from build123d import *

# Parameters (mm, degrees)
SKETCH2_R           = 0.635
BOSS_EXTRUDE1_DEPTH = 4.5
CIRPATTERN1_COUNT   = 4
CIRPATTERN1_ANGLE   = 216


with BuildPart() as part:
    # Sketch1 → Revolve1 (revolve)
    with BuildSketch(Plane.XY, mode=Mode.PRIVATE) as revolve1_sk:
        Polygon((0, 0), (7.6, 0), (7.6, -2.3), (6.375, -2.3), (6.375, -15.8), (5.728350463, -15.8), (5.728350463, -20.8), (0, -20.8), align=None)
    revolve(revolve1_sk.sketch.rotate(Axis((0, -20.8, 0), (0, 1, 0)), 90), axis=Axis((0, -20.8, 0), (0, 1, 0)))

    # Sketch2 → Boss-Extrude1 (add)
    with BuildSketch(Plane.XZ.offset(20.8)):
        with Locations(Location((0, 3.773128742, 0), (0, 0, 270))):
            Circle(SKETCH2_R)
    boss_extrude1 = extrude(amount=BOSS_EXTRUDE1_DEPTH)

    # CirPattern1: Boss-Extrude1 ×4 about axis
    cirpattern1_axis = Axis((0, 0, 0), (0, -1, 0))
    for i in range(1, CIRPATTERN1_COUNT):
        add(boss_extrude1.rotate(cirpattern1_axis, i * CIRPATTERN1_ANGLE / (CIRPATTERN1_COUNT - 1)))


solid = part.part
Source: CAD feature listing. Evaluate the final solid. Frame: model axes, mm. A direction names the side the tool comes from. Coordinates: 2 decimals unless noted, no trailing zeros. Loops run counter-clockwise (first coordinate to the right, second up) from the corner with the lowest first, then second, coordinate; pieces in that order, holes last. Notation, with made-up numbers: (42.25, 45) - (47.25, 45) arc R12 ccw to (47.25, 50) - close; hole circle Ø11 at (4.5, -27). An arc over 180 degrees is marked (long way). One line per item, written item: value. Start each with the question number.
1. Section B-B (x = 0). Return the cut outline in (y, z) (3 decimals), and give its area (3 significant figures).
2. Contact query for flat-ended pins moving along their axis: P1, Ø8, axis at x = 1.5, y = -17.5, coming from the +Z side (3 decimals); P2, Ø1, axis at x = -5.5, y = -4.5, coming from the -Z side; P3, Ø4, axis at y = -6.5, z = 2.5, coming from the -X side. Output: stop coordinate, or through.
3. Ray query, L1, parallel to Y at x = -1.5, z = -3.25; L2, parallel to Y at x = -6.5, z = 3.5; L3, parallel to X at y = -9.5, z = 0.25. Return the intervals inside material, ascending.
4. Set-up query: faces 1 (the flat face through (0, -25.3, 4)), 2 (the flat face through (-1, -15.8, 6)). Return all of +Z, -Z, +X, -X, +Y, -Y with unobstructed straight access to the full face (end or side cutting, diameter ignored); none if empty.
5. Section D-D (y = -22). Return the cut outline in (x, z) (3 decimals), and give its area (3 significant figures).
6. Section A-A (z = 0). Return the cut outline in (x, y) (3 decimals), and give its area (3 significant figures).
7. Mould query, pull axis X, two halves, no side actions, for faces 3 (the cylindrical face through (3.486, -18.335, 4.546)), 4 (the cylindrical face through (1.71, -23.02, -2.67)), 5 (the cylindrical face through (-2.02, -23.02, -2.45)), 6 (the flat face through (-4, -25.3, 1)). Classes: pulls with the +X half, pulls with the -X half, needs draft (parallel to the pull), parting line crosses it, or undercut.
8. Section C-C (y = -9.5). Return the cut outline in (x, z) (3 decimals), and give its area (3 significant figures).
Verdict:
1. outline: (-25.3, 3.138) - (-20.8, 3.138) - (-20.8, -5.728) - (-15.8, -5.728) - (-15.8, -6.375) - (-2.3, -6.375) - (-2.3, -7.6) - (0, -7.6) - (0, 7.6) - (-2.3, 7.6) - (-2.3, 6.375) - (-15.8, 6.375) - (-15.8, 5.728) - (-20.8, 5.728) - (-20.8, 4.408) - (-25.3, 4.408) - close
1. area: 270 mm2
2. P1: stops at z = 6.375
2. P2: stops at z = -3.95
2. P3: stops at x = -6.36
3. L1: y = -20.8 to 0
3. L2: y = -2.3 to 0
3. L3: x = -6.37 to 6.37
4. face 1: +Z, -Z, +X, -X, -Y
4. face 2: -Y
5. outline: circle Ø1.27 at (-3.588, 1.166); circle Ø1.27 at (-2.218, -3.053); circle Ø1.27 at (0, 3.773); circle Ø1.27 at (2.218, -3.053)
5. area: 5.07 mm2
6. outline: (-7.6, -2.3) - (-6.375, -2.3) - (-6.375, -15.8) - (-5.728, -15.8) - (-5.728, -20.8) - (5.728, -20.8) - (5.728, -15.8) - (6.375, -15.8) - (6.375, -2.3) - (7.6, -2.3) - (7.6, 0) - (-7.6, 0) - close
6. area: 264 mm2
7. face 3: parting line crosses it
7. face 4: undercut
7. face 5: undercut
7. face 6: needs draft
8. outline: circle Ø12.75 at (0, 0)
8. area: 128 mm2
